For this review, take the finished solid that the model builds, in its own axes (mm). Face numbers are marked on the shaded views. A direction names the side the tool comes from. Give positions to 0.01 mm unless a question says otherwise; leave off trailing zeros. Write each loop counter-clockwise with the first axis right and the second up, starting at its lowest first coordinate (ties: lowest second). Pieces come first, ordered by that corner, then holes. Notation, with made-up numbers: (41, -22) -> (52, -22) arc R16 cw to (52, 9) -> close; hole circle Ø2 at (14, 63). An arc over 180 degrees is marked (long way). Write item = value, one per line.
```python
from build123d import *

# Parameters (mm, degrees)
ESQUISSE1_W             = 0.5
ESQUISSE1_H             = 39
EXTRUSION1_DEPTH        = 13.5
ESQUISSE1_W_2           = 18.7
ESQUISSE1_H_2           = 0.5
EXTRUSION1_2_DEPTH      = 13.5
EXTRUSION1_3_DEPTH      = 13.5
EXTRUSION1_4_DEPTH      = 13.5
ESQUISSE2_W             = 19.9
ESQUISSE2_H             = 39
EXTRUSION2_DEPTH        = 0.5
ENL_V_MAT_EXTRU_1_DEPTH = 10
ESQUISSE4_W             = 1
ESQUISSE4_H             = 0.5
EXTRUSION3_DEPTH        = 2
ESQUISSE5_R             = 2
ENL_V_MAT_EXTRU_2_DEPTH = 2


with BuildPart() as part:
    # Esquisse1 → Extrusion1 (new body)
    with BuildSketch(Plane.XY):
        with Locations((-80.79228109, 4.736105473)):
            Rectangle(ESQUISSE1_W, ESQUISSE1_H)
    extrude(amount=EXTRUSION1_DEPTH)



with BuildPart() as body_2:
    # Esquisse1 → Extrusion1 2 (new body)
    with BuildSketch(Plane.XY):
        with Locations((-71.09228109, 23.986105473)):
            Rectangle(ESQUISSE1_W_2, ESQUISSE1_H_2)
    extrude(amount=EXTRUSION1_2_DEPTH)


with BuildPart() as body_3:
    # Esquisse1 → Extrusion1 3 (new body)
    with BuildSketch(Plane.XY):
        with Locations((-61.39228109, 4.736105473)):
            Rectangle(ESQUISSE1_W, ESQUISSE1_H)
    extrude(amount=EXTRUSION1_3_DEPTH)


with BuildPart() as body_4:
    # Esquisse1 → Extrusion1 4 (new body)
    with BuildSketch(Plane.XY):
        with Locations((-71.09228109, -14.513894527)):
            Rectangle(ESQUISSE1_W_2, ESQUISSE1_H_2)
    extrude(amount=EXTRUSION1_4_DEPTH)


with BuildPart() as part_1:
    add(part.part)

    add(body_2.part)  # Extrusion2 merges body 2

    add(body_3.part)  # Extrusion2 merges body 3

    add(body_4.part)  # Extrusion2 merges body 4
    # Esquisse2 → Extrusion2 (add)
    with BuildSketch(Plane.XY.offset(13.5)):
        with Locations((-71.09228109, 4.736105473)):
            Rectangle(ESQUISSE2_W, ESQUISSE2_H)
    extrude(amount=EXTRUSION2_DEPTH)

    # Esquisse3 → Enlèv. mat.-Extru.1 (cut)
    with BuildSketch(Plane(origin=(-61.14228109, 0, 0), x_dir=(0, 0, -1), z_dir=(1, 0, 0))):
        with BuildLine():
            Line((0, 18.236105473), (0, 10.236105473))
            Line((0, 10.236105473), (-3.3, 10.236105473))
            ThreePointArc((-3.3, 10.236105473), (-7.3, 14.236105473), (-3.3, 18.236105473))
            Line((-3.3, 18.236105473), (0, 18.236105473))
        make_face()
    extrude(amount=-ENL_V_MAT_EXTRU_1_DEPTH, mode=Mode.SUBTRACT)

    # Esquisse4 → Extrusion3 (add)
    with BuildSketch(Plane(origin=(0, 0, 0), x_dir=(-1, 0, 0), z_dir=(0, 0, -1))):
        with Locations((63.59228109, 23.986105473)):
            Rectangle(ESQUISSE4_W, ESQUISSE4_H)
        with Locations((78.59228109, 23.986105473)):
            Rectangle(ESQUISSE4_W, ESQUISSE4_H)
        with Locations((63.59228109, -14.513894527)):
            Rectangle(ESQUISSE4_W, ESQUISSE4_H)
        with Locations((78.59228109, -14.513894527)):
            Rectangle(ESQUISSE4_W, ESQUISSE4_H)
    extrude(amount=EXTRUSION3_DEPTH)

    # Esquisse5 → Enlèv. mat.-Extru.2 (cut)
    with BuildSketch(Plane.XY.offset(14)):
        with Locations((-71.19228109, -4.248125646)):
            Circle(ESQUISSE5_R)
    extrude(amount=-ENL_V_MAT_EXTRU_2_DEPTH, mode=Mode.SUBTRACT)


solid = part_1.part
```
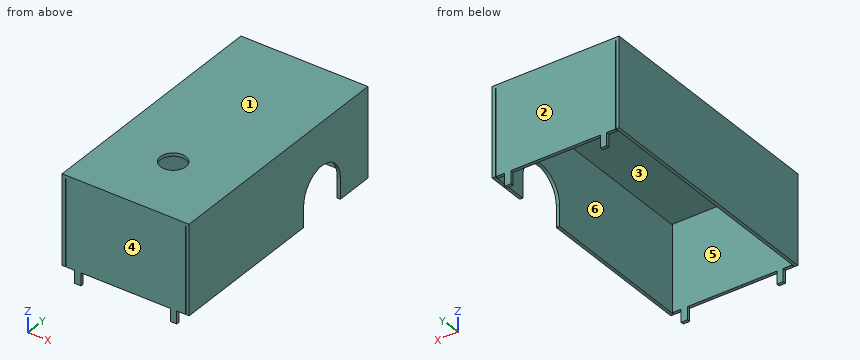
(1) Take a section at A-A (y = 22.5). Write out the cut boundary in (x, z), plus the area to 4 significant figures.
Answers below:
outline = (-81.04, 0) -> (-80.54, 0) -> (-80.54, 13.5) -> (-61.64, 13.5) -> (-61.64, 0) -> (-61.14, 0) -> (-61.14, 14) -> (-81.04, 14) -> close
area = 23.45 mm^2
(2) Take a section at C-C (x = -62.5). Write out the cut boundary in (y, z).
Answers below:
outline = (-14.76, 0) -> (-14.26, 0) -> (-14.26, 13.5) -> (23.74, 13.5) -> (23.74, 0) -> (24.24, 0) -> (24.24, 14) -> (-14.76, 14) -> close
(3) Tool access review of the marked faces 4, 5 and 6: name each direction out of +Z, -Z, +X, -X, +Y, -Y from which nothing blocks a thin tool from reaching the whole face with its end or side.
Answers below:
face_4 = +Z, -Z, +X, -X, -Y
face_5 = -Z
face_6 = -Z, +Y, -Y
(4) Take a section at D-D (x = -71). Write out the cut boundary in (y, z).
Answers below:
outline = (-14.76, 0) -> (-14.26, 0) -> (-14.26, 13.5) -> (-6.24, 13.5) -> (-6.24, 14) -> (-14.76, 14) -> close; (-2.26, 13.5) -> (23.74, 13.5) -> (23.74, 0) -> (24.24, 0) -> (24.24, 14) -> (-2.26, 14) -> close
(5) To check wall thickness, follow probe 1 along Y at (x, z) = (-75.25, 3); probe 2 along X at (y, z) = (-1, 10.5); probe 3 along Z at (x, y) = (-76.25, 15.5). State the ranges of each line that lie inside material, in increasing order.
Answers below:
probe_1 = -14.76 to -14.26, 23.74 to 24.24
probe_2 = -81.04 to -80.54, -61.64 to -61.14
probe_3 = 13.5 to 14
(6) The part is to be moulded in two halves that separate along Y. For the marked faces 1, 2 and 3, say which applies: released by +Y, released by -Y, zero draft, split by the parting line, or undercut.
Answers below:
face_1 = zero draft
face_2 = released by +Y
face_3 = undercut
(7) Take a section at B-B (z = 2.25). Write out the cut boundary in (x, y).
Answers below:
outline = (-81.04, -14.76) -> (-80.54, -14.76) -> (-80.54, 24.24) -> (-81.04, 24.24) -> close; (-80.44, -14.76) -> (-61.74, -14.76) -> (-61.74, -14.26) -> (-80.44, -14.26) -> close; (-80.44, 23.74) -> (-61.74, 23.74) -> (-61.74, 24.24) -> (-80.44, 24.24) -> close; (-61.64, -14.76) -> (-61.14, -14.76) -> (-61.14, 10.24) -> (-61.64, 10.24) -> close; (-61.64, 18.24) -> (-61.14, 18.24) -> (-61.14, 24.24) -> (-61.64, 24.24) -> close
(8) For pin 1 (1 mm diameter, centred on x = -73.5, y = -1, fed in from -Z); pin 2 (0.6 mm diameter, centred on x = -71, y = -14.5, fed in from -Z), all flat-tipped, find the tip position at first contact; note any pin that passes through.
Answers below:
pin_1 = 13.5
pin_2 = 0
